Could you check a few things on this model? Use its own coordinates, in mm. Coordinates: 2 decimals unless noted, no trailing zeros. Write each loop counter-clockwise with the first axis right and the second up, starting at its lowest first coordinate (ties: lowest second). Pieces come first, ordered by that corner, then holes. Notation, with made-up numbers: M 72,14 L 106,14 A11 ccw 106,25 Z; hole C 36.25,-24 d2. An arc over 180 degrees is marked long. Answer as CSV lines item,"result". Start each with the question number.
Item 1: If I drill on line 1 along Y through (x, z) = (19.5, 1.7); line 2 along Y through (x, z) = (21, 2.5); line 3 along Z through (x, y) = (-19, 17.5), over which ranges is the centre line in solid material (lowest first)? Write a range as [from, to].
Item 2: Suppose I cut it at A-A, the plane z = 0.8. Write out the boundary of the cut face in (x, y), and give its area (3 significant figures).
Item 3: Suppose I cut it at B-B, the plane y = -18.5. State how many separate pieces and enclosed holes the cut face has, and give its area (3 significant figures).
Item 4: We'd pull the mould along X, two halves only. Please class faces 1 (the cylindrical face through (18.21, 20.68, 2.19)), 2 (the flat face through (0, 25, 1)), 3 (the cylindrical face through (23.35, 23.43, 1.52)), 4 (the cylindrical face through (-23.43, 23.35, 1.52)): +X half, -X half, draft (parallel to the pull), parting line (faces both ways), or undercut.
Item 5: I'm going to push a flat-ended pin straight in: P1, Ø2, axis at x = -19.5, y = 19.5, coming from the -Z side. Where does the tip first touch, or does it pass through?
```python
from build123d import *

# Parameters (mm, degrees)
F0_W     = 50
F0_H     = 50
F0_R     = 1.75
F1_DEPTH = 3
F2_R     = 5.5
F3_SIZE  = 1.4


with BuildPart() as f1:
    # F0 (on Top) → F1 (new body)
    with BuildSketch(Plane.XY):
        Rectangle(F0_W, F0_H)
        with Locations((-19.5, -19.5)):
            Circle(F0_R, mode=Mode.SUBTRACT)
        with Locations((19.5, -19.5)):
            Circle(F0_R, mode=Mode.SUBTRACT)
        with Locations((-19.5, 19.5)):
            Circle(F0_R, mode=Mode.SUBTRACT)
        with Locations((19.5, 19.5)):
            Circle(F0_R, mode=Mode.SUBTRACT)
    extrude(amount=F1_DEPTH)

    # F2
    f2_edges = [f1.edges().sort_by_distance(p)[0] for p in [
        (-25, -25, 1.5),
        (25, -25, 1.5),
        (25, 25, 1.5),
        (-25, 25, 1.5),
    ]]
    fillet(f2_edges, radius=F2_R)

    # F3
    f3_edges = [f1.edges().sort_by_distance(p)[0] for p in [
        (-21.25, -19.5, 0),
        (-21.25, 19.5, 0),
        (17.75, 19.5, 0),
        (17.75, -19.5, 0),
    ]]
    chamfer(f3_edges, length=F3_SIZE)


solid = f1.part
```
Ans:
1,line 1,"y = [-25, -21.25], [-17.75, 17.75], [21.25, 25]"
1,line 2,"y = [-24.79, -20.4], [-18.6, 18.6], [20.4, 24.79]"
1,line 3,"z = [1.09, 3]"
2,outline,"M -25,-19.5 A5.5 ccw -19.5,-25 L 19.5,-25 A5.5 ccw 25,-19.5 L 25,19.5 A5.5 ccw 19.5,25 L -19.5,25 A5.5 ccw -25,19.5 Z; hole C -19.5,-19.5 d4.7; hole C -19.5,19.5 d4.7; hole C 19.5,-19.5 d4.7; hole C 19.5,19.5 d4.7"
2,area,"2,400 mm^2"
3,separate pieces,"3"
3,enclosed holes,"0"
3,area,"128 mm^2"
4,face 1,"undercut"
4,face 2,"draft"
4,face 3,"+X half"
4,face 4,"-X half"
5,P1,"passes through"
